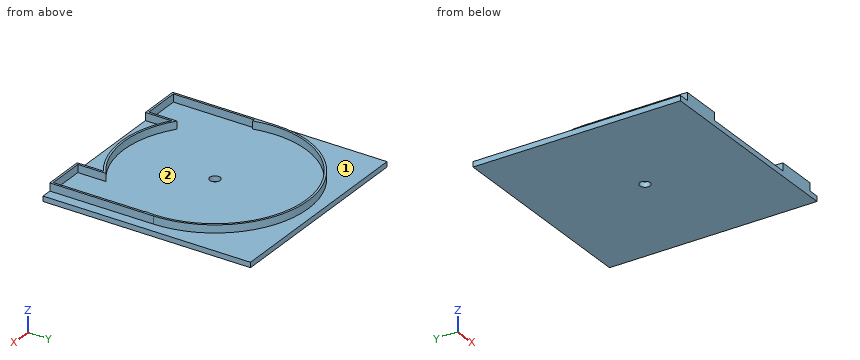
Autodesk Inventor part; units mm, degrees
ref_plane "YZ Plane" through (0, 0, 0) normal (1, 0, 0) x (0, 1, 0)
ref_plane "XZ Plane" through (0, 0, 0) normal (0, 1, 0) x (-1, 0, 0)
ref_plane "XY Plane" through (0, 0, 0) normal (0, 0, 1) x (1, 0, 0)
sketch "Sketch1" plane through (0, 0, 0) normal (0, 0, 1) x (1, 0, 0)
  line L0 (10, -10) -> (-10, -10)
  line L1 (-10, -10) -> (-10, 10)
  line L2 (-10, 10) -> (10, 10)
  line L3 (10, 10) -> (10, -10)
  line L4 (10, -10) -> (-10, 10) construction
  line L5 (-10, -10) -> (10, 10) construction
  point P0 (0, 0)
  dimension "d0" = 20
  dimension "d1" = 20
extrude "Extrusion1" add sketch "Sketch1" along normal blind 0.5
sketch "Sketch2" plane through (0, 0, 0.5) normal (0, 0, 1) x (1, 0, 0)
  point P0 (0, 0)
sketch "Sketch3" plane through (0, 0, 0.5) normal (0, 0, 1) x (1, 0, 0)
  line L0 (-10, -10) -> (10, -10)
  line L1 (-5, -7.4833) -> (-5, -10)
  line L2 (-5, -10) -> (-9, -10)
  line L3 (-9, -10) -> (-9, 0)
  line L4 (5, 0) -> (9, 0)
  line L5 (9, 0) -> (9, -10)
  line L6 (9, -10) -> (5, -10)
  line L7 (5, -10) -> (5, -7.4833)
  line L8 (-10, 10) -> (-10, -10)
  line L9 (10, -10) -> (10, 10)
  arc A0 (-5, -7.4833) -> (5, -7.4833) centre (0, 0) ccw
  arc A1 (9, 0) -> (-9, 0) centre (0, 0) ccw
  dimension "d4" = 4
  dimension "d5" = 1
  dimension "d6" = 1
extrude "Extrusion2" add sketch "Sketch3" along normal blind 0.75 contours L3 A1 L5 L0 L7 A0 L1
sketch "Sketch4" plane through (0, 0, 1.25) normal (0, 0, 1) x (1, 0, 0)
  line L0 (-8.8, -2) -> (-8.5697, -2)
  line L1 (-5.2, -7.0993) -> (-5.2, -9.8)
  line L2 (-5.2, -9.8) -> (-8.8, -9.8)
  line L3 (-8.8, -9.8) -> (-8.8, -2)
  line L4 (-9, 0) -> (-9, -10)
  line L5 (-9, -10) -> (-5, -10)
  line L6 (-5, -10) -> (-5, -7.4833)
  line L7 (8.743, -1) -> (8.8, -1)
  line L8 (8.8, -1) -> (8.8, -9.8)
  line L9 (8.8, -9.8) -> (5.2, -9.8)
  line L10 (5.2, -9.8) -> (5.2, -7.0993)
  line L11 (9, -10) -> (9, 0)
  line L12 (5, -10) -> (9, -10)
  line L13 (5, -7.4833) -> (5, -10)
  arc A0 (-5.2, -7.0993) -> (5.2, -7.0993) centre (0, 0) ccw
  arc A1 (8.743, -1) -> (-8.5697, -2) centre (0, 0) ccw
  dimension "d9" = 0.2
  dimension "d10" = 0.2
  dimension "d11" = 0.2
  dimension "d12" = 0.2
  dimension "d13" = 0.2
  dimension "d14" = 0.2
extrude "Extrusion3" cut sketch "Sketch4" against normal blind 0.75
sketch "Sketch6" plane through (0, 0, 0.5) normal (0, 0, 1) x (1, 0, 0)
  point P0 (0, 0)
sketch "Sketch9" plane through (0, 0, 0.5) normal (0, 0, 1) x (1, 0, 0)
  circle A0 centre (0, 0) radius 0.5
  dimension "d20" = 1
extrude "Extrusion5" cut sketch "Sketch9" against normal blind 0.5
properties part number "base" material "Aluminum 3004-H32"
Source: CAD feature listing. Evaluate the final solid. Frame: model axes, mm. Face numbers are marked on the shaded views. Give positions to 0.01 mm unless a question says otherwise; leave off trailing zeros. Loops run counter-clockwise (first coordinate to the right, second up) from the corner with the lowest first, then second, coordinate; pieces in that order, holes last. Notation, with made-up numbers: (-14, -7) -> (17, -7) arc R20 ccw to (17, 19) -> close; hole circle Ø3 at (-15, 60). An arc over 180 degrees is marked (long way). Use a Markdown table: item, result. Add a question column.
(1) Section query C-C (y = -3.25). Output: boundary loops of the cut face in (x, z).
(2) First-contact query: pin 1 Ø1 at (x, y) = (6, -6) entering from -Z; pin 2 Ø0.6 at (x, z) = (6, 1) entering from +Y; pin 3 Ø5.5 at (x, y) = (3.5, -1.5) entering from +Z. Flat tips, straight axial feed; report the tip coordinate or a pass-through.
(3) Section query D-D (x = -4.5). Output: boundary loops of the cut face in (y, z), then the cut area to 3 significant figures.
(4) Ray query, line 1 (Y direction, x = 0, z = 0.25); line 2 (Z direction, x = -6.25, y = -7); line 3 (X direction, y = 3, z = 0.55). Return the intervals inside material, ascending.
(5) Pull-direction query (Y, two-part tool) for the marked faces 1 and 2; classes: +Y half, -Y half, draft (parallel to the pull), parting line (faces both ways), or undercut.
(6) Section query B-B (z = 0.95). Output: boundary loops of the cut face in (x, y).
(7) Section query A-A (x = 0). Output: boundary loops of the cut face in (y, z).
Checked values:
| question | item | result |
|---|---|---|
| 1 | outline | (-10, 0) -> (10, 0) -> (10, 0.5) -> (9, 0.5) -> (9, 1.25) -> (8.8, 1.25) -> (8.8, 0.5) -> (-8.8, 0.5) -> (-8.8, 1.25) -> (-9, 1.25) -> (-9, 0.5) -> (-10, 0.5) -> close |
| 2 | pin 1 | z = 0 |
| 2 | pin 2 | y = 6.96 |
| 2 | pin 3 | z = 0.5 |
| 3 | outline | (-10, 0) -> (10, 0) -> (10, 0.5) -> (7.79, 0.5) -> (7.79, 1.25) -> (7.56, 1.25) -> (7.56, 0.5) -> (-7.56, 0.5) -> (-7.56, 1.25) -> (-7.79, 1.25) -> (-7.79, 0.5) -> (-10, 0.5) -> close |
| 3 | area | 10.3 mm^2 |
| 4 | line 1 | -10 to -0.5, 0.5 to 10 |
| 4 | line 2 | 0 to 0.5 |
| 4 | line 3 | -8.49 to -8.27, 8.27 to 8.49 |
| 5 | face 1 | draft |
| 5 | face 2 | undercut |
| 6 | outline | (-9, -10) -> (-5, -10) -> (-5, -7.48) arc R9 ccw to (5, -7.48) -> (5, -10) -> (9, -10) -> (9, 0) arc R9 ccw to (-9, 0) -> close; hole (-8.8, -9.8) -> (-5.2, -9.8) -> (-5.2, -7.1) arc R8.8 ccw to (5.2, -7.1) -> (5.2, -9.8) -> (8.8, -9.8) -> (8.8, -1) -> (8.74, -1) arc R8.8 ccw (long way) to (-8.57, -2) -> (-8.8, -2) -> close |
| 7 | outline | (-10, 0) -> (-0.5, 0) -> (-0.5, 0.5) -> (-8.8, 0.5) -> (-8.8, 1.25) -> (-9, 1.25) -> (-9, 0.5) -> (-10, 0.5) -> close; (0.5, 0) -> (10, 0) -> (10, 0.5) -> (9, 0.5) -> (9, 1.25) -> (8.8, 1.25) -> (8.8, 0.5) -> (0.5, 0.5) -> close |
